Answer from the drawing. Dimensions are ordinates in mm from the lowest x, y and z of the part. A direction names the side the tool comes from. Round coordinates to 2 decimals unless told otherwise and drop trailing zeros. Write each loop counter-clockwise with the first axis right and the second up, starting at its lowest first coordinate (ties: lowest second). Pieces come first, ordered by that corner, then holes. Notation, with made-up numbers: M -14.5,-26.5 L 10.5,-26.5 A19 ccw 10.5,-13.5 Z; hole C 49,-40 d9. An arc over 180 degrees is marked long. One line per item, written item: value. Start each with the question number.
(1) Consider probe 1 along Y at (x, z) = (13.75, 3.35); probe 2 along Y at (x, z) = (20.25, 1.1) (1 decimal); probe 3 along X at (y, z) = (11.25, 2.1). Determine where each line is inside the solid, lowest interval first.
(2) For a pull along Y with two mould halves and no side action, classify the marked faces 1, 2 and 3 as released by +Y, released by -Y, zero draft, split by the parting line, or undercut.
(3) Section D-D (z = 3.15) is taken. Determine the outline of the cut face in (x, y).
(4) Given P1, Ø1.5, axis at x = 11.5, z = 3, coming from the -Y side; P2, Ø1.5, axis at y = 8.5, z = 1, coming from the +X side; P3, Ø1.5, axis at y = 9.5, z = 0.5, coming from the -X side, each flat-ended and moving along its own axis, determine where each tip first touches the part or whether it passes through.
(5) Section B-B (z = 0.9) is taken. State how many separate pieces and enclosed holes the cut face has, plus the area to 3 significant figures.
(6) For the marked faces 4, 5 and 6, determine the directions among +Z, -Z, +X, -X, +Y, -Y from which every point of the face is accessible in a straight line to the end or side of a thin tool.
(7) Section C-C (y = 16.5) is taken. Determine the outline of the cut face in (x, z).
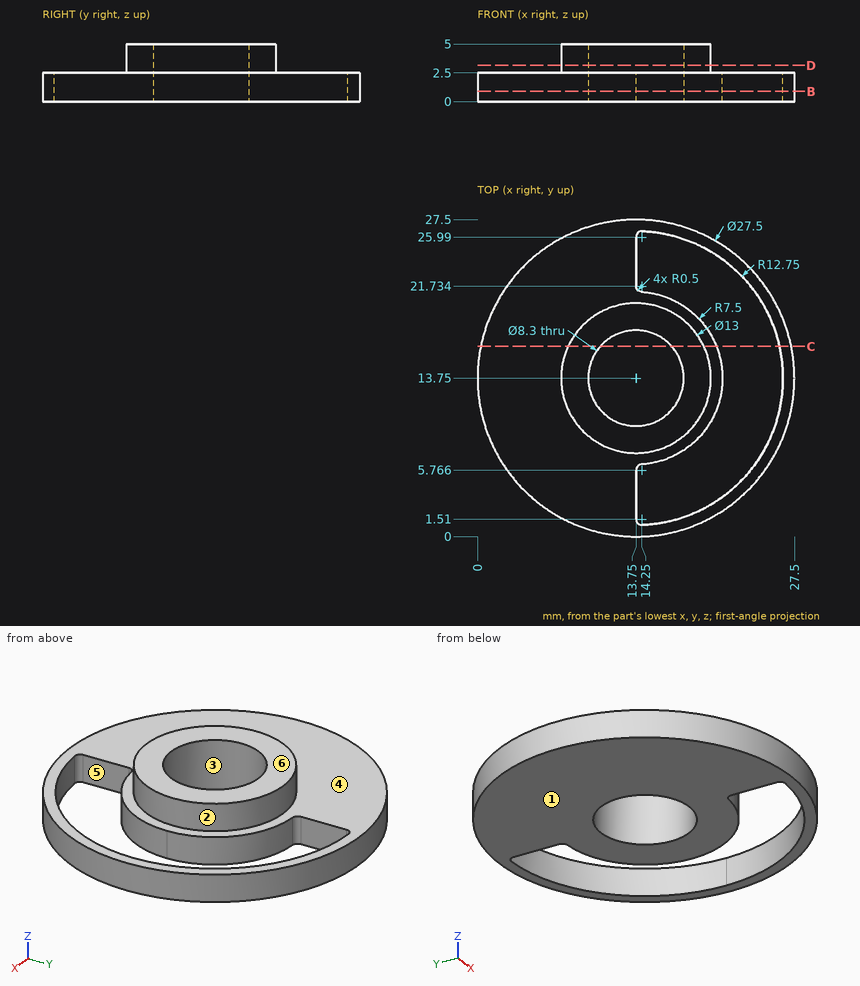
Recorded:
1. probe 1: y = 7.25 to 9.6, 17.9 to 20.25
1. probe 2: y = 1.6 to 2.8, 10 to 17.5, 24.7 to 25.9
1. probe 3: x = 0.23 to 10.44, 17.06 to 20.82, 26.25 to 27.27
2. face 1: zero draft
2. face 2: split by the parting line
2. face 3: undercut
3. outline: C 13.75,13.75 d13; hole C 13.75,13.75 d8.3
4. P1: stops at y = 0.1
4. P2: stops at x = 26.74
4. P3: stops at x = 0.45
5. separate pieces: 1
5. enclosed holes: 2
5. area: 373 mm2
6. face 4: +Z
6. face 5: +Z, -Z
6. face 6: +Z, +X, -X, +Y, -Y
7. outline: M 0.28,0 L 10.64,0 L 10.64,5 L 7.86,5 L 7.86,2.5 L 0.28,2.5 Z; M 16.86,0 L 20.73,0 L 20.73,2.5 L 19.64,2.5 L 19.64,5 L 16.86,5 Z; M 26.2,0 L 27.22,0 L 27.22,2.5 L 26.2,2.5 Z
